Source: CAD feature listing. Evaluate the final solid. Frame: model axes, mm. A direction names the side the tool comes from. Give positions to 0.01 mm unless a question says otherwise; leave off trailing zeros. Loops run counter-clockwise (first coordinate to the right, second up) from the corner with the lowest first, then second, coordinate; pieces in that order, holes last. Notation, with made-up numbers: (6, -10.5) -> (47, -10.5) arc R32 ccw to (47, 17.5) -> close; hole circle Ø11 at (21, -12.75). An arc over 180 degrees is marked (long way). Answer as a JSON object with one key per item and string values. Group by question number.
from build123d import *

# Parameters (mm, degrees)
SKETCH2_R           = 115
BOSS_EXTRUDE1_DEPTH = 3
SKETCH3_R           = 112
BOSS_EXTRUDE2_DEPTH = 3
SKETCH4_R           = 98
BOSS_EXTRUDE3_DEPTH = 93
SKETCH5_R           = 95
CUT_EXTRUDE1_DEPTH  = 96
SKETCH6_R           = 35
BOSS_EXTRUDE4_DEPTH = 100
SKETCH7_R           = 32
BOSS_EXTRUDE5_DEPTH = 5
SKETCH8_R           = 32
CUT_EXTRUDE2_DEPTH  = 99
SKETCH9_R           = 28
CUT_EXTRUDE3_DEPTH  = 4
SKETCH10_R          = 10
BOSS_EXTRUDE8_DEPTH = 5
SKETCH11_R          = 7
CUT_EXTRUDE4_DEPTH  = 35
SKETCH13_W          = 25
SKETCH13_H          = 13
CUT_EXTRUDE5_DEPTH  = 10
SKETCH14_W          = 15
SKETCH14_H          = 3
CUT_EXTRUDE7_DEPTH  = 10


with BuildPart() as part:
    # Sketch2 → Boss-Extrude1 (new body)
    with BuildSketch(Plane(origin=(0, 0, 0), x_dir=(1, 0, 0), z_dir=(0, 1, 0))):
        with Locations(Location((0, 0, 0), (0, 0, 270))):
            Circle(SKETCH2_R)
    extrude(amount=BOSS_EXTRUDE1_DEPTH)

    # Sketch3 → Boss-Extrude2 (add)
    with BuildSketch(Plane(origin=(0, 0, 0), x_dir=(-1, 0, 0), z_dir=(0, -1, 0))):
        with Locations(Location((0, 0, 0), (0, 0, 90))):
            Circle(SKETCH3_R)
    extrude(amount=BOSS_EXTRUDE2_DEPTH)

    # Sketch4 → Boss-Extrude3 (add)
    with BuildSketch(Plane.XZ.offset(3)):
        with Locations(Location((0, 0, 0), (0, 0, 270))):
            Circle(SKETCH4_R)
    extrude(amount=BOSS_EXTRUDE3_DEPTH)

    # Sketch5 → Cut-Extrude1 (cut)
    with BuildSketch(Plane(origin=(0, 3, 0), x_dir=(1, 0, 0), z_dir=(0, 1, 0))):
        with Locations(Location((0, 0, 0), (0, 0, 270))):
            Circle(SKETCH5_R)
    extrude(amount=-CUT_EXTRUDE1_DEPTH, mode=Mode.SUBTRACT)

    # Sketch6 → Boss-Extrude4 (add)
    with BuildSketch(Plane(origin=(0, -93, 0), x_dir=(1, 0, 0), z_dir=(0, 1, 0))):
        with Locations(Location((0, 0, 0), (0, 0, 270))):
            Circle(SKETCH6_R)
    extrude(amount=BOSS_EXTRUDE4_DEPTH)

    # Sketch7 → Boss-Extrude5 (add)
    with BuildSketch(Plane(origin=(0, 7, 0), x_dir=(1, 0, 0), z_dir=(0, 1, 0))):
        with Locations(Location((0, 0, 0), (0, 0, 270))):
            Circle(SKETCH7_R)
    extrude(amount=BOSS_EXTRUDE5_DEPTH)

    # Sketch8 → Cut-Extrude2 (cut)
    with BuildSketch(Plane.XZ.offset(96)):
        with Locations(Location((0, 0, 0), (0, 0, 90))):
            Circle(SKETCH8_R)
    extrude(amount=-CUT_EXTRUDE2_DEPTH, mode=Mode.SUBTRACT)

    # Sketch9 → Cut-Extrude3 (cut)
    with BuildSketch(Plane.XZ.offset(-3)):
        with Locations(Location((0, 0, 0), (0, 0, 270))):
            Circle(SKETCH9_R)
    extrude(amount=-CUT_EXTRUDE3_DEPTH, mode=Mode.SUBTRACT)

    # Sketch10 → Boss-Extrude8 (add)
    with BuildSketch(Plane(origin=(0, 12, 0), x_dir=(1, 0, 0), z_dir=(0, 1, 0))):
        with Locations(Location((0, 0, 0), (0, 0, 270))):
            Circle(SKETCH10_R)
    extrude(amount=BOSS_EXTRUDE8_DEPTH)

    # Sketch11 → Cut-Extrude4 (cut)
    with BuildSketch(Plane(origin=(0, 17, 0), x_dir=(1, 0, 0), z_dir=(0, 1, 0))):
        with Locations(Location((0, 0, 0), (0, 0, 270))):
            Circle(SKETCH11_R)
    extrude(amount=-CUT_EXTRUDE4_DEPTH, mode=Mode.SUBTRACT)

    # Sketch13 → Cut-Extrude5 (cut)
    with BuildSketch(Plane(origin=(0, 10, 0), x_dir=(1, 0, 0), z_dir=(0, 1, 0))):
        with Locations((0, -104.95033264)):
            Rectangle(SKETCH13_W, SKETCH13_H)
    extrude(amount=-CUT_EXTRUDE5_DEPTH, mode=Mode.SUBTRACT)

    # Sketch14 → Cut-Extrude7 (cut)
    with BuildSketch(Plane(origin=(0, 0, 0), x_dir=(1, 0, 0), z_dir=(0, 1, 0))):
        with Locations((0, -101.95033264)):
            Rectangle(SKETCH14_W, SKETCH14_H)
    extrude(amount=-CUT_EXTRUDE7_DEPTH, mode=Mode.SUBTRACT)


solid = part.part
(1) Material intervals for line 1 (X direction, y = -40, z = 0); line 2 (X direction, y = 12.75, z = 0); line 3 (Z direction, x = -18, y = -31), sorted ascending. Write a range as from..to.
(2) Section query A-A on y = -50. Return the cut outline in (x, z), plus the area to 3 significant figures.
(3) Mould query, pull axis Z, two halves, no side actions, for faces 4 (the face through (-92.74, -44.33, -20.59)), 5 (the face through (-28.4, 7, 15.4)), 6 (the face through (29.437, -48.849, -93.475)). Classes: pulls with the +Z half, pulls with the -Z half, needs draft (parallel to the pull), parting line crosses it, or undercut.
(4) Section query B-B on x = 0. State how many separate pieces and enclosed holes the cut face has, plus the area to 3 significant figures.
(5) Access query for faces 1 (the face through (-112.265, 1.479, -24.93)), 2 (the face through (-6, 7, -6)), 3 (the face through (0, 0, 105)). Directions: +Z, -Z, +X, -X, +Y, -Y. A direction counts if a zero-diameter tool reaches every point of the face in a straight line with its end or side. Return the directions, or none.
(6) First-contact query: pin 1 (6.5 mm diameter, centred on x = 6, z = 108, fed in from +Y); pin 2 (0.9 mm diameter, centred on x = 2.5, y = 1.5, fed in from -Z); pin 3 (3 mm diameter, centred on y = 1.5, z = -30.5, fed in from -X). Flat tips, straight axial feed; report the tip coordinate or a pass-through.
(7) Section query C-C on z = -81. Return the cut outline in (x, y).
(8) Section query D-D on x = -71. Return the cut outline in (y, z).
Result:
{
 "1": {"line 1": "-98..-95, -35..-32, 32..35, 95..98", "line 2": "-10..-7, 7..10", "line 3": "-96.33..-93.28, -30.02..-26.46, 26.46..30.02, 93.28..96.33"},
 "2": {"outline": "circle Ø196 at (0, 0); circle Ø70 at (0, 0); hole circle Ø190 at (0, 0); hole circle Ø64 at (0, 0)", "area": "2,450 mm²"},
 "3": {"face 4": "undercut", "face 5": "needs draft", "face 6": "parting line crosses it"},
 "4": {"separate pieces": "3", "enclosed holes": "0", "area": "2,020 mm²"},
 "5": {"face 1": "+Y, -Y", "face 2": "-Y", "face 3": "+Y"},
 "6": {"pin 1": "y = 0", "pin 2": "z = -114.98", "pin 3": "x = -111.28"},
 "7": {"outline": "(-81.63, 0) -> (-77.35, 0) -> (-77.35, -3) -> (-55.16, -3) -> (-55.16, -96) -> (55.16, -96) -> (55.16, -3) -> (77.35, -3) -> (77.35, 0) -> (81.63, 0) -> (81.63, 3) -> (49.64, 3) -> (49.64, -93) -> (-49.64, -93) -> (-49.64, 3) -> (-81.63, 3) -> close"},
 "8": {"outline": "(-96, -67.55) -> (-3, -67.55) -> (-3, -86.62) -> (0, -86.62) -> (0, -90.47) -> (3, -90.47) -> (3, -63.12) -> (-93, -63.12) -> (-93, 63.12) -> (3, 63.12) -> (3, 90.47) -> (0, 90.47) -> (0, 86.62) -> (-3, 86.62) -> (-3, 67.55) -> (-96, 67.55) -> close"}
}
